Design review of the part built by this model. Coordinates are the model's own, in mm. Face numbers are marked on the shaded views. A direction names the side the tool comes from. Coordinates: 2 decimals unless noted, no trailing zeros. Order: outer loops, then holes, each group sorted by start corner. A loop starts at its lowest first (then second) coordinate and runs counter-clockwise, first axis right, second up.
from build123d import *

# Parameters (mm, degrees)
BOSS_EXTRU_1_DEPTH      = 15
ESQUISSE2_W             = 42
ESQUISSE2_H             = 22
ENL_V_MAT_EXTRU_1_DEPTH = 48.360320945
ESQUISSE4_R             = 2.15
ENL_V_MAT_EXTRU_2_DEPTH = 3
ESQUISSE5_W             = 4
ESQUISSE5_H             = 6.35
ENL_V_MAT_EXTRU_3_DEPTH = 6
ESQUISSE6_W             = 4
ESQUISSE6_H             = 6.35
ENL_V_MAT_EXTRU_4_DEPTH = 8
BOSS_EXTRU_2_DEPTH      = 5
BOSS_EXTRU_2_DEPTH_BACK = 5
CHANFREIN1_SIZE         = 3
BOSS_EXTRU_4_DEPTH      = 5
BOSS_EXTRU_6_START      = 20
ESQUISSE13_W            = 12.5
ESQUISSE13_H            = 10
BOSS_EXTRU_6_DEPTH      = 20
ESQUISSE14_W            = 42
ESQUISSE14_H            = 10
BOSS_EXTRU_7_DEPTH      = 5
BOSS_EXTRU_8_START      = -5
BOSS_EXTRU_8_DEPTH      = 5
ESQUISSE17_R            = 4.5
ENL_V_MAT_EXTRU_5_DEPTH = 130.352109985


with BuildPart() as part:
    # Esquisse1 → Boss.-Extru.1 (new body)
    with BuildSketch(Plane.XY):
        with BuildLine():
            Line((30, -13), (-30, -13))
            Line((-30, -13), (-30, 13))
            Line((-30, 13), (30, 13))
            ThreePointArc((30, 13), (43, 0), (30, -13))
        make_face()
    extrude(amount=BOSS_EXTRU_1_DEPTH)

    # Esquisse2 → Enlèv. mat.-Extru.1 (cut, through all)
    with BuildSketch(Plane.XY.offset(15)):
        with Locations((3, 0)):
            Rectangle(ESQUISSE2_W, ESQUISSE2_H)
    extrude(amount=-ENL_V_MAT_EXTRU_1_DEPTH, mode=Mode.SUBTRACT)

    # Esquisse4 → Enlèv. mat.-Extru.2 (cut)
    with BuildSketch(Plane.XY.offset(15)):
        with Locations((-20.81, 4.935)):
            Circle(ESQUISSE4_R)
        with Locations((-20.81, -4.935)):
            Circle(ESQUISSE4_R)
        with Locations((28.49, 4.935)):
            Circle(ESQUISSE4_R)
        with Locations((28.49, -4.935)):
            Circle(ESQUISSE4_R)
    extrude(amount=-ENL_V_MAT_EXTRU_2_DEPTH, mode=Mode.SUBTRACT)

    # Esquisse5 → Enlèv. mat.-Extru.3 (cut)
    with BuildSketch(Plane(origin=(-18, 0, 0), x_dir=(0, 0, -1), z_dir=(1, 0, 0))):
        with Locations((-10, -4.825)):
            Rectangle(ESQUISSE5_W, ESQUISSE5_H)
        with Locations((-10, 4.825)):
            Rectangle(ESQUISSE5_W, ESQUISSE5_H)
    extrude(amount=-ENL_V_MAT_EXTRU_3_DEPTH, mode=Mode.SUBTRACT)

    # Esquisse6 → Enlèv. mat.-Extru.4 (cut)
    with BuildSketch(Plane.ZY.offset(-24)):
        with Locations((10, 4.825)):
            Rectangle(ESQUISSE6_W, ESQUISSE6_H)
        with Locations((10, -4.825)):
            Rectangle(ESQUISSE6_W, ESQUISSE6_H)
    extrude(amount=-ENL_V_MAT_EXTRU_4_DEPTH, mode=Mode.SUBTRACT)

    # Esquisse9 → Boss.-Extru.2 (add, two sides: drawn at the far end of the back side and taken through both)
    with BuildSketch(Plane.XY.offset(7.5).offset(-BOSS_EXTRU_2_DEPTH_BACK)):
        Polygon((-30, -33), (-30, 33), (-95, 33), (-95, 28), (-35, 28), (-35, -28), (-95, -28), (-95, -33), align=None)
    extrude(amount=BOSS_EXTRU_2_DEPTH + BOSS_EXTRU_2_DEPTH_BACK)

    # Chanfrein1
    # the kernel refuses this chamfer: 3 mm, written as the material it adds along each edge
    with BuildSketch(Plane(origin=(-30, -13, 12.5), x_dir=(0.02749587661058678, 0, 0.9996219169112968), z_dir=(0, 1, 0))) as chanfrein1_piece_1_section:
        Polygon((CHANFREIN1_SIZE * 0.999621916911, -CHANFREIN1_SIZE * 0.0274958766106), (-CHANFREIN1_SIZE * 0.0274958766106, -CHANFREIN1_SIZE * 0.999621916911), (0, 0), align=None)
    chanfrein1_piece_1 = extrude(amount=26, mode=Mode.PRIVATE)
    chanfrein1_piece_1 = split(chanfrein1_piece_1, bisect_by=Plane(origin=(-31.023809524, 0, 15), z_dir=(0, 0, -1)), keep=Keep.TOP, mode=Mode.PRIVATE)
    add(chanfrein1_piece_1)
    with BuildSketch(Plane(origin=(-30, -13, 2.5), x_dir=(0.027495876610586778, 0, -0.9996219169112968), z_dir=(0, 1, 0))) as chanfrein1_piece_2_section:
        Polygon((CHANFREIN1_SIZE * 0.999621916911, CHANFREIN1_SIZE * 0.0274958766106), (-CHANFREIN1_SIZE * 0.0274958766106, CHANFREIN1_SIZE * 0.999621916911), (0, 0), align=None)
    chanfrein1_piece_2 = extrude(amount=26, mode=Mode.PRIVATE)
    chanfrein1_piece_2 = split(chanfrein1_piece_2, bisect_by=Plane(origin=(-31.023809524, 0, 0), z_dir=(0, 0, 1)), keep=Keep.TOP, mode=Mode.PRIVATE)
    add(chanfrein1_piece_2)

    # Esquisse11 → Boss.-Extru.4 (add)
    with BuildSketch(Plane.XZ.offset(33)):
        with BuildLine():
            Line((-95, 2.5), (-95, 12.5))
            Line((-95, 12.5), (-104.43476759, 12.5))
            ThreePointArc((-104.43476759, 12.5), (-109.43476759, 7.5), (-104.43476759, 2.5))
            Line((-104.43476759, 2.5), (-95, 2.5))
        make_face()
    extrude(amount=-BOSS_EXTRU_4_DEPTH)

    # Esquisse13 → Boss.-Extru.6 (add)
    with BuildSketch(Plane(origin=(0, 0, 0), x_dir=(-1, 0, 0), z_dir=(0, 0, -1)).offset(BOSS_EXTRU_6_START)):
        with BuildLine():
            Line((-24, -5), (-24, 5))
            Line((-24, 5), (-42, 5))
            ThreePointArc((-42, 5), (-43, 0), (-42, -5))
            Line((-42, -5), (-24, -5))
        make_face()
        with Locations((24.25, 0)):
            Rectangle(ESQUISSE13_W, ESQUISSE13_H)
    extrude(amount=-BOSS_EXTRU_6_DEPTH)

    # Esquisse14 → Boss.-Extru.7 (add)
    with BuildSketch(Plane(origin=(0, 0, -20), x_dir=(-1, 0, 0), z_dir=(0, 0, -1))):
        with Locations((-3, 0)):
            Rectangle(ESQUISSE14_W, ESQUISSE14_H)
    extrude(amount=-BOSS_EXTRU_7_DEPTH)

    # Esquisse16 → Boss.-Extru.8 (add)
    with BuildSketch(Plane(origin=(0, 33, 0), x_dir=(1, 0, 0), z_dir=(0, 1, 0)).offset(BOSS_EXTRU_8_START)):
        with BuildLine():
            Line((-89.416041875, -12.5), (-104.43476759, -12.5))
            ThreePointArc((-104.43476759, -12.5), (-109.43476759, -7.5), (-104.43476759, -2.5))
            Line((-104.43476759, -2.5), (-89.416041875, -2.5))
            Line((-89.416041875, -2.5), (-89.416041875, -12.5))
        make_face()
    extrude(amount=BOSS_EXTRU_8_DEPTH)

    # Esquisse17 → Enlèv. mat.-Extru.5 (cut, through all)
    with BuildSketch(Plane.XZ.offset(33)):
        with Locations((-95, 7.5)):
            Circle(ESQUISSE17_R)
    extrude(amount=-ENL_V_MAT_EXTRU_5_DEPTH, mode=Mode.SUBTRACT)


solid = part.part
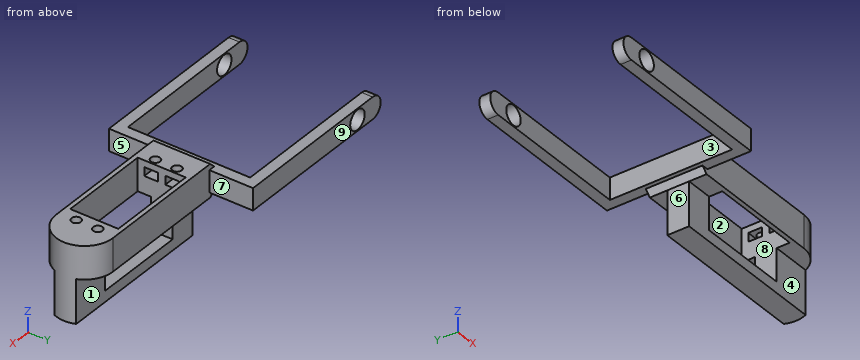
1. Mouldability with a two-part tool opening along X and no side actions: class the marked faces 6, 7, 8 and 9 as pulls with the +X half, pulls with the -X half, needs draft (parallel to the pull), parting line crosses it, or undercut.
2. Add section C-C (x = -9.5). Give the boundary of the cut face in (y, z).
3. Add section D-D (x = 28.49). Give the boundary of the cut face in (y, z) (3 decimals).
4. Add section B-B (y = 0). Give the boundary of the cut face in (x, z), and give its area (3 significant figures).
5. Add section A-A (x = -87). Give the boundary of the cut face in (y, z), and give its area (3 significant figures).
6. To check wall thickness, follow line 1 (Y direction, x = 17, z = 12); line 2 (Z direction, x = -95, y = -29); line 3 (Y direction, x = -64, z = 7). State the ranges of each line that lie inside material, in increasing order.
7. For the marked faces 1, 2, 3, 4 and 5, list the 3-axis set-ups (+Z, -Z, +X, -X, +Y, -Y) from which the entire face can be reached by the end or side of a thin tool; tool diameter is ignored.
8. Insertion check: pin 1 (2 mm diameter, centred on x = -19.5, z = 10.5, fed in from +Y); pin 2 (6 mm diameter, centred on x = -0.5, z = 9.5, fed in from -Y); pin 3 (4 mm diameter, centred on y = -3, z = 11.5, fed in from -X). Each pin has a flat end and moves straight along its axis. Give the tip position at first contact, or say it passes through.
Solution:
1. face 6: pulls with the -X half
1. face 7: pulls with the +X half
1. face 8: undercut
1. face 9: needs draft
2. outline: (-13, 0) - (-11, 0) - (-11, 15) - (-13, 15) - close; (-5, -20) - (5, -20) - (5, -15) - (-5, -15) - close; (11, 0) - (13, 0) - (13, 15) - (11, 15) - close
3. outline: (-13, 0) - (-5, 0) - (-5, -20) - (5, -20) - (5, 0) - (13, 0) - (13, 15) - (7.085, 15) - (7.085, 12) - (8, 12) - (8, 8) - (1.65, 8) - (1.65, 12) - (2.785, 12) - (2.785, 15) - (-2.785, 15) - (-2.785, 12) - (-1.65, 12) - (-1.65, 8) - (-8, 8) - (-8, 12) - (-7.085, 12) - (-7.085, 15) - (-13, 15) - close
4. outline: (-35, 2.5) - (-33, 2.5) - (-30.5, 0) - (-30.5, -20) - (43, -20) - (43, 15) - (24, 15) - (24, -15) - (-18, -15) - (-18, 15) - (-30.5, 15) - (-33, 12.5) - (-35, 12.5) - close
4. area: 1,360 mm2
5. outline: (-33, 2.5) - (-28, 2.5) - (-28, 12.5) - (-33, 12.5) - close; (28, 2.5) - (33, 2.5) - (33, 12.5) - (28, 12.5) - close
5. area: 100 mm2
6. line 1: y = -13 to -11, 11 to 13
6. line 2: z = 2.5 to 3, 12 to 12.5
6. line 3: y = -33 to -28, 28 to 33
7. face 1: -Z, +X, -X, +Y
7. face 2: +Z, -Z
7. face 3: +Z, -Z, -X
7. face 4: -Z, +X, -X, -Y
7. face 5: +Z, -Z, +X, -Y
8. pin 1: stops at y = 13
8. pin 2: stops at y = -13
8. pin 3: stops at x = -35
